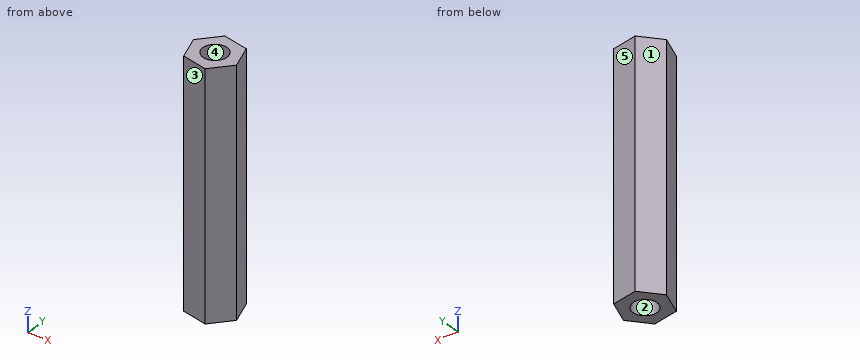
Autodesk Inventor part; units mm, degrees
ref_plane "YZ Plane" through (0, 0, 0) normal (1, 0, 0) x (0, 1, 0)
ref_plane "XZ Plane" through (0, 0, 0) normal (0, 1, 0) x (-1, 0, 0)
ref_plane "XY Plane" through (0, 0, 0) normal (0, 0, 1) x (1, 0, 0)
sketch "スケッチ1" plane through (0, 0, 0) normal (0, 0, 1) x (1, 0, 0)
  circle A0 centre (0, 0) radius 3
  circle A1 centre (0, 0) radius 1.5
  line L0 (2.0761, 2.4027) -> (3.1189, -0.5966)
  line L1 (3.1189, -0.5966) -> (1.0427, -2.9993)
  line L2 (1.0427, -2.9993) -> (-2.0761, -2.4027)
  line L3 (-2.0761, -2.4027) -> (-3.1189, 0.5966)
  line L4 (-3.1189, 0.5966) -> (-1.0427, 2.9993)
  line L5 (-1.0427, 2.9993) -> (2.0761, 2.4027)
  dimension "d0" = 6
  dimension "d1" = 3
  dimension "d13" = 5.5
extrude "押し出し1" add sketch "スケッチ1" along normal blind 30 contours L0 A0 L1 L2 L3 L4 L5 | A0 L5 L0 | L0 L1 A0 | A0 L4 L5 | L1 L2 A0 | A0 L3 L4 | L2 L3 A0
thread "ねじ1"
extrude "押し出し2" add sketch "スケッチ1" along normal blind 24 contours A1
extrude "押し出し3" cut sketch "スケッチ1" along normal blind 6 contours A1
thread "ねじ2"
properties part number "スペーサーM3L30樹脂" material "PBT プラスチック"
Work out the finished part from the listing and answer in its coordinate system (mm). Face numbers are marked on the shaded views. A direction names the side the tool comes from. Coordinates: 2 decimals unless noted, no trailing zeros. Write each loop counter-clockwise with the first axis right and the second up, starting at its lowest first coordinate (ties: lowest second). Pieces come first, ordered by that corner, then holes.
Q1. A cutting plane is placed at D-D, the plane z = 11. Give the vertices of the cut face in (x, y).
Q2. A cutting plane is placed at B-B, the plane y = 0.9. Give the vertices of the cut face in (x, z), then the cut area to 3 significant figures.
Q3. Determine the mould class of the marked faces 3, 4 and 5 for opening direction X: released by +X, released by -X, zero draft, split by the parting line, or undercut.
Q4. Which of the six approach directions +Z, -Z, +X, -X, +Y, -Y give full straight-line access (tool end or side, diameter ignored) to the marked faces 1 and 2?
Q5. A cutting plane is placed at C-C, the plane x = 0. Give the vertices of the cut face in (y, z), then the cut area to 3 significant figures.
Q6. Find the intervals of material crossed by line 1 (Z direction, x = 1.25, y = -0.6); line 2 (Y direction, x = 0, z = 25.6); line 3 (Y direction, x = 0.5, z = 4.5), in increasing order.
Q7. Each of these flat-tipped pins is pushed along its axis until it touches: pin 1 Ø2.5 at (x, y) = (0, 0) entering from +Z; pin 2 Ø0.9 at (x, y) = (-0.5, 0.5) entering from -Z; pin 3 Ø1.5 at (x, z) = (-2, 17) entering from +Y. Where does it stop, or does it pass through?
Q8. A cutting plane is placed at A-A, the plane z = 3.75. Give the vertices of the cut face in (x, y), then the cut area to 3 significant figures.
Findings below:
1. outline: (-3.12, 0.6) - (-2.08, -2.4) - (1.04, -3) - (3.12, -0.6) - (2.08, 2.4) - (-1.04, 3) - close
2. outline: (-2.86, 0) - (-1.2, 0) - (-1.2, 6) - (1.2, 6) - (1.2, 0) - (2.6, 0) - (2.6, 30) - (1.2, 30) - (1.2, 24) - (-1.2, 24) - (-1.2, 30) - (-2.86, 30) - close
2. area: 135 mm2
3. face 3: released by -X
3. face 4: undercut
3. face 5: released by +X
4. face 1: +Z, -Z, -X, +Y
4. face 2: -Z
5. outline: (-2.8, 0) - (-1.5, 0) - (-1.5, 6) - (1.5, 6) - (1.5, 0) - (2.8, 0) - (2.8, 30) - (1.5, 30) - (1.5, 24) - (-1.5, 24) - (-1.5, 30) - (-2.8, 30) - close
5. area: 132 mm2
6. line 1: z = 6 to 24
6. line 2: y = -2.8 to -1.5, 1.5 to 2.8
6. line 3: y = -2.9 to -1.41, 1.41 to 2.7
7. pin 1: stops at z = 24
7. pin 2: stops at z = 6
7. pin 3: stops at y = 2.76
8. outline: (-3.12, 0.6) - (-2.08, -2.4) - (1.04, -3) - (3.12, -0.6) - (2.08, 2.4) - (-1.04, 3) - close; hole circle Ø3 at (0, 0)
8. area: 19.1 mm2
